Can you work these out from the model? Positions are in its coordinate system, mm. A direction names the side the tool comes from. Give positions to 0.01 mm unless a question says otherwise; leave off trailing zeros. Order: outer loops, then holes, each group sorted by start corner. A loop starts at its lowest first (then second) coordinate and runs counter-clockwise, first axis right, second up. Notation, with made-up numbers: (73.25, 86.5) - (132.25, 86.5) arc R15 cw to (132.25, 109.5) - close; hole circle Ø11 at (4.5, 72). An arc over 180 degrees is marked (long way). Answer as CSV lines item,"result".
```python
from build123d import *

# Parameters (mm, degrees)
ESQUISSE1_W                  = 62
ESQUISSE1_H                  = 30
BOSS_EXTRU_1_DEPTH           = 18
ENL_V_MAT_EXTRU_1_DEPTH      = 72.189886922
ENL_V_MAT_EXTRU_1_DEPTH_BACK = 72.189886922
ESQUISSE2_R                  = 12.8
ENL_V_MAT_EXTRU_2_DEPTH      = 72.189886922
ENL_V_MAT_EXTRU_2_DEPTH_BACK = 72.189886922
ESQUISSE3_W                  = 15
ESQUISSE3_H                  = 3
ENL_V_MAT_EXTRU_3_DEPTH      = 72.189886922
ENL_V_MAT_EXTRU_3_DEPTH_BACK = 72.189886922
ESQUISSE4_R                  = 6.45
ESQUISSE4_R_2                = 3.25
ENL_V_MAT_EXTRU_4_DEPTH      = 72.189886922
ENL_V_MAT_EXTRU_4_DEPTH_BACK = 72.189886922
ESQUISSE6_W                  = 15
ESQUISSE6_H                  = 3
ENL_V_MAT_EXTRU_5_DEPTH      = 72.189886922
ENL_V_MAT_EXTRU_5_DEPTH_BACK = 72.189886922
ESQUISSE8_R                  = 3.25
ESQUISSE9_R                  = 4.25
ENL_V_MAT_EXTRU_6_DEPTH      = 12.7
ESQUISSE10_R                 = 4.25
ENL_V_MAT_EXTRU_7_DEPTH      = 6
CHANFREIN1_SIZE              = 0.5
CHANFREIN2_SIZE              = 1


with BuildPart() as part:
    # Esquisse1 → Boss.-Extru.1 (new body)
    with BuildSketch(Plane.XY):
        with Locations((31, 15)):
            Rectangle(ESQUISSE1_W, ESQUISSE1_H)
    extrude(amount=BOSS_EXTRU_1_DEPTH)

    # Esquisse2 → Enlèv. mat.-Extru.1 (cut, two sides: drawn at the far end of the back side and taken through both)
    with BuildSketch(Plane.XY.offset(18).offset(-ENL_V_MAT_EXTRU_1_DEPTH_BACK)):
        with Locations((24, 15)):
            Circle(ESQUISSE2_R)
    extrude(amount=ENL_V_MAT_EXTRU_1_DEPTH + ENL_V_MAT_EXTRU_1_DEPTH_BACK, mode=Mode.SUBTRACT)

    # Esquisse3 → Enlèv. mat.-Extru.2 (cut, two sides: drawn at the far end of the back side and taken through both)
    with BuildSketch(Plane.XY.offset(18).offset(-ENL_V_MAT_EXTRU_2_DEPTH_BACK)):
        with Locations((7.5, 15)):
            Rectangle(ESQUISSE3_W, ESQUISSE3_H)
    extrude(amount=ENL_V_MAT_EXTRU_2_DEPTH + ENL_V_MAT_EXTRU_2_DEPTH_BACK, mode=Mode.SUBTRACT)

    # Esquisse4 → Enlèv. mat.-Extru.3 (cut, two sides: drawn at the far end of the back side and taken through both)
    with BuildSketch(Plane.XZ.offset(-ENL_V_MAT_EXTRU_3_DEPTH_BACK)):
        with Locations(Location((45, 9, 0), (0, 0, 270))):
            Circle(ESQUISSE4_R)
        with Locations((6, 9)):
            Circle(ESQUISSE4_R_2)
    extrude(amount=ENL_V_MAT_EXTRU_3_DEPTH + ENL_V_MAT_EXTRU_3_DEPTH_BACK, mode=Mode.SUBTRACT)

    # Esquisse6 → Enlèv. mat.-Extru.4 (cut, two sides: drawn at the far end of the back side and taken through both)
    with BuildSketch(Plane.XZ.offset(-ENL_V_MAT_EXTRU_4_DEPTH_BACK)):
        with Locations((54.5, 9)):
            Rectangle(ESQUISSE6_W, ESQUISSE6_H)
    extrude(amount=ENL_V_MAT_EXTRU_4_DEPTH + ENL_V_MAT_EXTRU_4_DEPTH_BACK, mode=Mode.SUBTRACT)

    # Esquisse8 → Enlèv. mat.-Extru.5 (cut, two sides: drawn at the far end of the back side and taken through both)
    with BuildSketch(Plane.XY.offset(18).offset(-ENL_V_MAT_EXTRU_5_DEPTH_BACK)):
        with Locations((56, 15)):
            Circle(ESQUISSE8_R)
    extrude(amount=ENL_V_MAT_EXTRU_5_DEPTH + ENL_V_MAT_EXTRU_5_DEPTH_BACK, mode=Mode.SUBTRACT)

    # Esquisse9 → Enlèv. mat.-Extru.6 (cut)
    with BuildSketch(Plane(origin=(0, 30, 0), x_dir=(1, 0, 0), z_dir=(0, 1, 0))):
        with Locations(Location((6, -9, 0), (0, 0, 270))):
            Circle(ESQUISSE9_R)
    extrude(amount=-ENL_V_MAT_EXTRU_6_DEPTH, mode=Mode.SUBTRACT)

    # Esquisse10 → Enlèv. mat.-Extru.7 (cut)
    with BuildSketch(Plane(origin=(0, 0, 0), x_dir=(-1, 0, 0), z_dir=(0, 0, -1))):
        with Locations((-56, 15)):
            Circle(ESQUISSE10_R)
    extrude(amount=-ENL_V_MAT_EXTRU_7_DEPTH, mode=Mode.SUBTRACT)

    # Chanfrein1
    # the kernel refuses this chamfer: 0.675653437, 0.570826882, 0.5 mm, written as the material it takes off along each edge
    with BuildSketch(Plane(origin=(6, 0, 9), x_dir=(1, 0, 0), z_dir=(0, 0, -1))) as chanfrein1_piece_1:
        Polygon((3.25 + CHANFREIN1_SIZE, 0), (3.25, -CHANFREIN1_SIZE), (3.25, 0), align=None)
    revolve(axis=Axis((6, 0, 9), (0, -1, 0)), mode=Mode.SUBTRACT)
    with BuildSketch(Plane(origin=(56, 15, 18), x_dir=(1, 0, 0), z_dir=(0, -1, 0))) as chanfrein1_piece_2:
        Polygon((3.25 + CHANFREIN1_SIZE, 0), (3.25, -CHANFREIN1_SIZE), (3.25, 0), align=None)
    revolve(axis=Axis((56, 15, 18), (0, 0, 1)), mode=Mode.SUBTRACT)
    with BuildSketch(Plane(origin=(6, 30, 9), x_dir=(0, 0, 1), z_dir=(-1, 0, 0))) as chanfrein1_piece_3:
        Polygon((4.25 + CHANFREIN1_SIZE, 0), (4.25, -CHANFREIN1_SIZE), (4.25, 0), align=None)
    revolve(axis=Axis((6, 30, 9), (0, 1, 0)), mode=Mode.SUBTRACT)
    with BuildSketch(Plane(origin=(56, 15, 0), x_dir=(-1, 0, 0), z_dir=(0, -1, 0))) as chanfrein1_piece_4:
        Polygon((4.25 + CHANFREIN1_SIZE, 0), (4.25, -CHANFREIN1_SIZE), (4.25, 0), align=None)
    revolve(axis=Axis((56, 15, 0), (0, 0, -1)), mode=Mode.SUBTRACT)
    with BuildSketch(Plane(origin=(11.288194463, 16.5, -1.516273716), x_dir=(0.1399712439743316, 0.990155569019474, 0), z_dir=(0, 0, 1))) as chanfrein1_piece_5:
        with BuildLine():
            Line((0.588107761, 0), (-CHANFREIN1_SIZE * 0.139971243974, CHANFREIN1_SIZE * 0.990155569019))
            Line((-CHANFREIN1_SIZE * 0.139971243974, CHANFREIN1_SIZE * 0.990155569019), (0, 0))
            ThreePointArc((0, 0), (0.303184371, 0.003374833), (0.588107761, 0))
        make_face()
    extrude(amount=21.032547433, mode=Mode.SUBTRACT)
    with BuildSketch(Plane(origin=(11.288194463, 13.5, -1.516273716), x_dir=(-1, 0, 0), z_dir=(0, 0, 1))) as chanfrein1_piece_6:
        with BuildLine():
            Line((CHANFREIN1_SIZE, 0), (-0.082318175, 0.582318175))
            ThreePointArc((-0.082318175, 0.582318175), (-0.039095484, 0.300672073), (0, 0))
            Line((0, 0), (CHANFREIN1_SIZE, 0))
        make_face()
    extrude(amount=21.032547433, mode=Mode.SUBTRACT)
    with BuildSketch(Plane(origin=(51.2731571, 31.928380981, 10.5), x_dir=(1, 0, 0), z_dir=(0, -1, 0))) as chanfrein1_piece_7:
        with BuildLine():
            Line((CHANFREIN1_SIZE, 0), (-0.215649634, 0.715649634))
            ThreePointArc((-0.215649634, 0.715649634), (-0.100904588, 0.372377882), (0, 0))
            Line((0, 0), (CHANFREIN1_SIZE, 0))
        make_face()
    extrude(amount=33.856761963, mode=Mode.SUBTRACT)
    with BuildSketch(Plane(origin=(51.2731571, 31.928380981, 7.5), x_dir=(-0.28851956060345535, 0, -0.9574740012915176), z_dir=(0, -1, 0))) as chanfrein1_piece_8:
        with BuildLine():
            Line((0.747435056, 0), (-CHANFREIN1_SIZE * 0.288519560603, CHANFREIN1_SIZE * 0.957474001292))
            Line((-CHANFREIN1_SIZE * 0.288519560603, CHANFREIN1_SIZE * 0.957474001292), (0, 0))
            ThreePointArc((0, 0), (0.385655089, 0.010824783), (0.747435056, 0))
        make_face()
    extrude(amount=33.856761963, mode=Mode.SUBTRACT)
    # the kernel refuses this chamfer: 0.675653437, 0.570826882, 0.5 mm, written as the material it takes off along each edge
    with BuildSketch(Plane(origin=(24, 15, 18), x_dir=(-0.9980557123023516, 0.06232812479648115, 0), z_dir=(-0.06232812479648115, -0.9980557123023516, 0))) as chanfrein1_2_piece_1:
        Polygon((12.8, CHANFREIN1_SIZE), (12.8 + CHANFREIN1_SIZE, 0), (12.8, 0), align=None)
    revolve(axis=Axis((24, 15, 18), (0, 0, -1)), revolution_arc=352.853090525, mode=Mode.SUBTRACT)
    with BuildSketch(Plane(origin=(24, 15, 0), x_dir=(-0.9980557123023512, -0.06232812479648351, 0), z_dir=(-0.06232812479648351, 0.9980557123023512, 0))) as chanfrein1_2_piece_2:
        Polygon((12.8, CHANFREIN1_SIZE), (12.8 + CHANFREIN1_SIZE, 0), (12.8, 0), align=None)
    revolve(axis=Axis((24, 15, 0), (0, 0, 1)), revolution_arc=352.853090525, mode=Mode.SUBTRACT)
    with BuildSketch(Plane(origin=(45, 30, 9), x_dir=(0.9887286551586735, 0, -0.14971855752751953), z_dir=(0.14971855752751953, 0, 0.9887286551586735))) as chanfrein1_2_piece_3:
        Polygon((6.45 + CHANFREIN1_SIZE, 0), (6.45, -CHANFREIN1_SIZE), (6.45, 0), align=None)
    revolve(axis=Axis((45, 30, 9), (0, 1, 0)), revolution_arc=342.778766173, mode=Mode.SUBTRACT)
    with BuildSketch(Plane(origin=(45, 0, 9), x_dir=(0.9887286551586734, 0, -0.14971855752752006), z_dir=(0.14971855752752006, 0, 0.9887286551586734))) as chanfrein1_2_piece_4:
        Polygon((6.45 + CHANFREIN1_SIZE, 0), (6.45, CHANFREIN1_SIZE), (6.45, 0), align=None)
    revolve(axis=Axis((45, 0, 9), (0, 1, 0)), revolution_arc=342.778766173, mode=Mode.SUBTRACT)

    # Chanfrein2
    chanfrein2_edges = [part.edges().sort_by_distance(p)[0] for p in [
        (62, 15, 18),
        (31, 30, 18),
        (0, 6.75, 0),
        (0, 6.75, 18),
        (0, 13.5, 9),
        (0, 16.5, 9),
        (0, 23.25, 18),
        (31, 30, 0),
        (62, 15, 0),
        (31, 0, 0),
        (62, 30, 3.75),
        (0, 23.25, 0),
        (62, 0, 3.75),
        (31, 0, 18),
        (0, 30, 9),
        (62, 30, 14.25),
        (62, 0, 14.25),
        (0, 0, 9),
    ]]
    chamfer(chanfrein2_edges, length=CHANFREIN2_SIZE)


solid = part.part
```
1) Which directions (+Z, -Z, +X, -X, +Y, -Y) give clear straight access to the entire face, cutting with the end or side of a thin tool? Please do faces 4 (the flat face through (2.6, 13.5, 8.9)), 5 (the flat face through (57, 19, 10.5)), 6 (the flat face through (31, 30, 9)).
Answer block:
face 4,"+Z, -Z, -X"
face 5,"+X, +Y, -Y"
face 6,"+Z, -Z, +X, -X, +Y"
2) I want a section at A-A on x = 24. Write out the boundary of the cut face in (y, z).
Answer block:
outline,"(0, 1) - (1, 0) - (1.7, 0) - (2.2, 0.5) - (2.2, 17.5) - (1.7, 18) - (1, 18) - (0, 17) - close; (27.8, 0.5) - (28.3, 0) - (29, 0) - (30, 1) - (30, 17) - (29, 18) - (28.3, 18) - (27.8, 17.5) - close"
3) I'm going to push a flat-ended pin straight in: P1, Ø2.5, axis at x = 4.5, z = 7, coming from the +Y side. Where does the tip first touch, or does it pass through?
Answer block:
P1,"y = 17.3"
4) I need wall thicknesses on line 1 along Y through (x, z) = (56, 3.7); line 2 along X through (y, z) = (18.5, 4); line 3 along Z through (x, y) = (53, 6). Which ranges of each line are inside material? Lowest first, please. Write a range as [from, to].
Answer block:
line 1,"[0, 10.75], [19.25, 30]"
line 2,"[0, 11.69], [36.31, 40.93], [49.07, 53.59], [58.41, 62]"
line 3,"[0, 7.5], [10.5, 18]"
5) If we mould it in two halves opening along Z, with no side actions, what happens to faces 1 (the flat face through (37.2, 18.3, 0)), 2 (the flat face through (31, 0, 9)), 3 (the cylindrical face through (3.41, 23.49, 5.63))? For each: +Z half, -Z half, draft (parallel to the pull), parting line (faces both ways), or undercut.
Answer block:
face 1,"-Z half"
face 2,"draft"
face 3,"undercut"
6) I want a section at B-B on x = 6. Write out the boundary of the cut face in (y, z).
Answer block:
outline,"(0, 1) - (1, 0) - (13.5, 0) - (13.5, 5.75) - (0.5, 5.75) - (0, 5.25) - close; (0, 12.75) - (0.5, 12.25) - (13.5, 12.25) - (13.5, 18) - (1, 18) - (0, 17) - close; (16.5, 0) - (29, 0) - (30, 1) - (30, 4.25) - (29.5, 4.75) - (17.3, 4.75) - (17.3, 5.75) - (16.5, 5.75) - close; (16.5, 12.25) - (17.3, 12.25) - (17.3, 13.25) - (29.5, 13.25) - (30, 13.75) - (30, 17) - (29, 18) - (16.5, 18) - close"
7) I want a section at C-C on y = 6.5. Count the separate pieces of the cut face and the enclosed holes in it, plus the area to 3 significant figures.
Answer block:
separate pieces,"2"
enclosed holes,"1"
area,"573 mm2"
8) I want a section at D-D on x = 45. Write out the boundary of the cut face in (y, z), plus the area to 4 significant figures.
Answer block:
outline,"(0, 1) - (1, 0) - (29, 0) - (30, 1) - (30, 2.05) - (29.5, 2.55) - (0.5, 2.55) - (0, 2.05) - close; (0, 15.95) - (0.5, 15.45) - (29.5, 15.45) - (30, 15.95) - (30, 17) - (29, 18) - (1, 18) - (0, 17) - close"
area,"150.5 mm2"
